Input: part model. Units: mm. Frame: model coordinates. A direction names the side the tool comes from. Give positions to 0.01 mm unless a question says otherwise; leave off trailing zeros. Loops run counter-clockwise (first coordinate to the right, second up) from the corner with the lowest first, then second, coordinate; pieces in that order, holes last. Notation, with made-up numbers: M 16,74.25 L 39,74.25 A8 ccw 39,87.25 Z; hole C 39.25,-26.75 d8. An arc over 180 degrees is marked long. Use CSV: the item, a comma, the result in double quotes. Start each with the question number.
Q1. Section C-C, the plane x = -3. Output: boundary loops of the cut face in (y, z), plus the area to 3 significant figures.
Q2. Material intervals for line 1 along Y through (x, z) = (-1.25, 0.65); line 2 along X through (y, z) = (-1.25, 0.3); line 3 along Y through (x, z) = (-4.5, 0.85), sorted ascending.
Q3. Section A-A, the plane y = 0. Output: boundary loops of the cut face in (x, z).
Q4. Pull-direction query (Y, two-part tool) for faces 1 (the flat face through (1.26, -3.46, 0.7)), 2 (the flat face through (2.368, 2.822, 0.695)), 3 (the cylindrical face through (-1.88, -5.02, 0.68)); classes: released by +Y, released by -Y, zero draft, split by the parting line, or undercut.
Q5. Reachability of faces 4 (the flat face through (-3.23, -1.865, 0.695)), 5 (the cylindrical face through (0.693, 1.933, 0.695)), 6 (the cylindrical face through (1.328, -1.567, 0.695)) from +Z, -Z, +X, -X, +Y, -Y: full face, straight path, thin tool, end or side. Return the list, or none.
Q6. Section B-B, the plane z = 0.55. Output: boundary loops of the cut face in (x, y).
Q7. Section D-D, the plane x = 4.25. Output: boundary loops of the cut face in (y, z), plus the area to 3 significant figures.
from build123d import *

# Parameters (mm, degrees)
F0_R      = 28.3757796524
F1_DEPTH  = 8.636
F2_R      = 3.772916628
F3_DEPTH  = 25.4
F5_R      = 5.3605373526
F6_DEPTH  = 1.3716
F7_R      = 1.4989937
F8_DEPTH  = 25.4
F10_DEPTH = 25.4


with BuildPart() as f1:
    # F0 (on Top) → F1 (new body)
    with BuildSketch(Plane.XY):
        with Locations((-28.4617077559, 15.6847797334)):
            Circle(F0_R)
    extrude(amount=F1_DEPTH)

    # F2 (on face) → F3 (cut)
    with BuildSketch(Plane.XY.offset(8.636)):
        with Locations((-28.4617077559, 15.6847797334)):
            Circle(F2_R)
    extrude(amount=-F3_DEPTH, mode=Mode.SUBTRACT)


with BuildPart() as f6:
    # F5 (on Top) → F6 (new body)
    with BuildSketch(Plane.XY):
        Circle(F5_R)
    extrude(amount=F6_DEPTH)

    # F7 (on face) → F8 (cut)
    with BuildSketch(Plane.XY.offset(1.3716)):
        Circle(F7_R)
    extrude(amount=-F8_DEPTH, mode=Mode.SUBTRACT)

    # F9 (on face) → F10 (cut)
    with BuildSketch(Plane.XY.offset(1.3716)):
        with BuildLine():
            Line((4.6423615252, -2.6802686763), (1.7784824816, -1.0268073395))
            ThreePointArc((1.7784824816, -1.0268073395), (1.3200380707, -1.5731601132), (0.7023775868, -1.9297665598))
            Line((0.7023775868, -1.9297665598), (1.8334117536, -5.0372573936))
            ThreePointArc((1.8334117536, -5.0372573936), (3.4456869915, -4.1064098511), (4.6423615252, -2.6802686763))
        make_face()
        with BuildLine():
            Line((-4.6423615252, -2.6802686763), (-1.7784824816, -1.0268073395))
            ThreePointArc((-1.7784824816, -1.0268073395), (-2.0224156576, -0.3566064466), (-2.0224156576, 0.3566064466))
            Line((-2.0224156576, 0.3566064466), (-5.2790987451, 0.9308475426))
            ThreePointArc((-5.2790987451, 0.9308475426), (-5.2790987451, -0.9308475426), (-4.6423615252, -2.6802686763))
        make_face()
        with BuildLine():
            ThreePointArc((0, 2.053614679), (0.7023775868, 1.9297665598), (1.3200380707, 1.5731601132))
            Line((1.3200380707, 1.5731601132), (3.4456869915, 4.1064098511))
            ThreePointArc((3.4456869915, 4.1064098511), (1.8334117536, 5.0372573936), (0, 5.3605373526))
            Line((0, 5.3605373526), (0, 2.053614679))
        make_face()
    extrude(amount=-F10_DEPTH, mode=Mode.SUBTRACT)


solid = f6.part
A:
1,outline,"M -4.44,0 L -1.73,0 L -1.73,1.37 L -4.44,1.37 Z; M 0.53,0 L 4.44,0 L 4.44,1.37 L 0.53,1.37 Z"
1,area,"9.09 mm^2"
2,line 1,"-5.21 to -0.83, 0.83 to 5.21"
2,line 2,"-2.17 to -0.83, 0.83 to 1.63, 2.17 to 5.21"
2,line 3,"-2.91 to -2.6, 0.79 to 2.91"
3,outline,"M -2.05,0 L -1.5,0 L -1.5,1.37 L -2.05,1.37 Z; M 1.5,0 L 5.36,0 L 5.36,1.37 L 1.5,1.37 Z"
4,face 1,"undercut"
4,face 2,"released by +Y"
4,face 3,"released by -Y"
5,face 4,"+Z, -Z, -X"
5,face 5,"+Z, -Z, +Y"
5,face 6,"+Z, -Z"
6,outline,"M -5.28,0.93 L -2.02,0.36 A2.05 ccw -1.78,-1.03 L -4.64,-2.68 A5.36 ccw 1.83,-5.04 L 0.7,-1.93 A2.05 ccw 1.78,-1.03 L 4.64,-2.68 A5.36 ccw 3.45,4.11 L 1.32,1.57 A2.05 ccw 0,2.05 L 0,5.36 A5.36 ccw Z; hole C 0,0 d3"
7,outline,"M -2.45,0 L 3.27,0 L 3.27,1.37 L -2.45,1.37 Z"
7,area,"7.85 mm^2"
